```python
from build123d import *

# Parameters (mm, degrees)
CROQUIS1_R              = 3.645
SALIENTE_EXTRUIR1_DEPTH = 26.3


with BuildPart() as part:
    # Croquis1 → Saliente-Extruir1 (new body)
    with BuildSketch(Plane(origin=(0, 0, 0), x_dir=(0, 0, -1), z_dir=(1, 0, 0))):
        with BuildLine():
            Line((-14.240976213, -40.83193708), (-9.515976213, -40.83193708))
            Line((-9.515976213, -40.83193708), (-15.665976213, -34.68193708))
            Line((-15.665976213, -34.68193708), (-23.665976213, -34.68193708))
            Line((-23.665976213, -34.68193708), (-29.815976213, -40.83193708))
            Line((-29.815976213, -40.83193708), (-25.090976213, -40.83193708))
            ThreePointArc((-25.090976213, -40.83193708), (-23.665976213, -42.25693708), (-25.090976213, -43.68193708))
            Line((-25.090976213, -43.68193708), (-33.267411985, -43.655501308))
            ThreePointArc((-33.267411985, -43.655501308), (-34.256346235, -43.245871329), (-34.665976213, -42.25693708))
            Line((-34.665976213, -42.25693708), (-34.665976213, -34.10693708))
            ThreePointArc((-34.665976213, -34.10693708), (-33.267411985, -32.708372853), (-31.868847758, -34.10693708))
            Line((-31.868847758, -34.10693708), (-31.868847758, -38.83193708))
            Line((-31.868847758, -38.83193708), (-25.718847758, -32.68193708))
            Line((-25.718847758, -32.68193708), (-25.718847758, -24.68193708))
            Line((-25.718847758, -24.68193708), (-31.868847758, -18.53193708))
            Line((-31.868847758, -18.53193708), (-31.868847758, -23.25693708))
            ThreePointArc((-31.868847758, -23.25693708), (-33.293847758, -24.68193708), (-34.718847758, -23.25693708))
            Line((-34.718847758, -23.25693708), (-34.718847758, -15.10698367))
            ThreePointArc((-34.718847758, -15.10698367), (-34.301474921, -14.099356507), (-33.293847758, -13.68198367))
            Line((-33.293847758, -13.68198367), (-25.143847758, -13.68198367))
            ThreePointArc((-25.143847758, -13.68198367), (-23.718847758, -15.10698367), (-25.143847758, -16.53198367))
            Line((-25.143847758, -16.53198367), (-29.868847758, -16.53198367))
            Line((-29.868847758, -16.53198367), (-23.718847758, -22.68198367))
            Line((-23.718847758, -22.68198367), (-15.718847758, -22.68198367))
            Line((-15.718847758, -22.68198367), (-9.568847758, -16.53198367))
            Line((-9.568847758, -16.53198367), (-14.293847758, -16.53198367))
            ThreePointArc((-14.293847758, -16.53198367), (-15.718847758, -15.10698367), (-14.293847758, -13.68198367))
            Line((-14.293847758, -13.68198367), (-6.143847758, -13.68198367))
            ThreePointArc((-6.143847758, -13.68198367), (-5.136220595, -14.099356507), (-4.718847758, -15.10698367))
            Line((-4.718847758, -15.10698367), (-4.718847758, -23.153239985))
            ThreePointArc((-4.718847758, -23.153239985), (-6.143847758, -24.578239985), (-7.568847758, -23.153239985))
            Line((-7.568847758, -23.153239985), (-7.568847758, -18.53198367))
            Line((-7.568847758, -18.53198367), (-13.718847758, -24.68198367))
            Line((-13.718847758, -24.68198367), (-13.718847758, -32.68198367))
            Line((-13.718847758, -32.68198367), (-7.568847758, -38.83198367))
            Line((-7.568847758, -38.83198367), (-7.568847758, -34.003239985))
            ThreePointArc((-7.568847758, -34.003239985), (-6.143847758, -32.578239985), (-4.718847758, -34.003239985))
            Line((-4.718847758, -34.003239985), (-4.718847758, -42.25693708))
            ThreePointArc((-4.718847758, -42.25693708), (-5.136220595, -43.264564244), (-6.143847758, -43.68193708))
            Line((-6.143847758, -43.68193708), (-14.240976213, -43.68193708))
            ThreePointArc((-14.240976213, -43.68193708), (-15.665976213, -42.25693708), (-14.240976213, -40.83193708))
        make_face()
        with Locations((-19.665976213, -28.68193708)):
            Circle(CROQUIS1_R, mode=Mode.SUBTRACT)
    extrude(amount=SALIENTE_EXTRUIR1_DEPTH)


solid = part.part
```
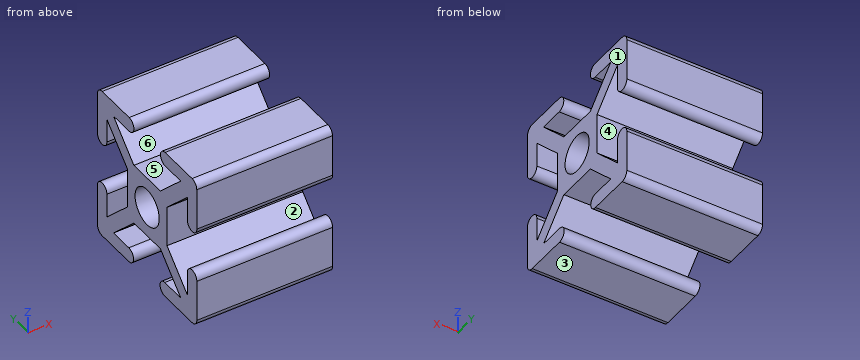
Build history of the part. All positions in model axes, mm. Face numbers are marked on the shaded views. A direction names the side the tool comes from. Round coordinates to 2 decimals unless told otherwise and drop trailing zeros. Loops run counter-clockwise (first coordinate to the right, second up) from the corner with the lowest first, then second, coordinate; pieces in that order, holes last.
Item 1: Drill centre lines: line 1 along Y through (x, z) = (7.5, 26); line 2 along Y through (x, z) = (10.75, 25); line 3 along Z through (x, y) = (12.25, -20.5). Where is each one in solid material? Low to high.
Item 2: Which spindle directions (+Z, -Z, +X, -X, +Y, -Y) get a long thin tool onto all of the face, cutting with end or side? Do the marked faces 4, 5 and 6. Say none if no direction does.
Item 3: Saw through at D-D (z = 27). List the corners of the cut face in (x, y), then the cut area to 3 significant figures.
Item 4: Saw through at A-A (y = -35.25). List the corners of the cut face in (x, z), then the cut area to 3 significant figures.
Item 5: Saw through at B-B (z = 15). List the corners of the cut face in (x, y).
Item 6: Saw through at C-C (z = 20.5). List the corners of the cut face in (x, y).
Item 7: Pin check, flat tips, straight feed: P1, Ø2.5, axis at x = 13, z = 27, coming from the -Y side; P2, Ø2.5, axis at x = 9.5, y = -38, coming from the +Z side; P3, Ø4, axis at x = 15, z = 20.5, coming from the -Y side. Stop position of each tip, or through.
Item 8: Two-plate mould, pull along Z, no slides. Class the marked faces 1, 2 and 3: released by +Z, released by -Z, zero draft, split by the parting line, or undercut.
Worked answers:
1. line 1: y = -43.68 to -40.83, -37.02 to -32.96, -24.4 to -20.4, -16.53 to -13.68
1. line 2: y = -43.68 to -40.83, -36.02 to -21.4, -16.52 to -13.69
1. line 3: z = 4.72 to 7.57, 9.54 to 13.54, 25.9 to 29.9, 31.87 to 34.72
2. face 4: +X, -X, +Y
2. face 5: +Z, +X, -X
2. face 6: +X, -X
3. outline: (0, -43.68) - (26.3, -43.68) - (26.3, -40.83) - (0, -40.83) - close; (0, -38.02) - (26.3, -38.02) - (26.3, -33.96) - (0, -33.96) - close; (0, -23.4) - (26.3, -23.4) - (26.3, -19.4) - (0, -19.4) - close; (0, -16.53) - (26.3, -16.53) - (26.3, -13.68) - (0, -13.68) - close
3. area: 362 mm2
4. outline: (0, 4.72) - (26.3, 4.72) - (26.3, 7.57) - (0, 7.57) - close; (0, 11.15) - (26.3, 11.15) - (26.3, 15.1) - (0, 15.1) - close; (0, 24.23) - (26.3, 24.23) - (26.3, 28.29) - (0, 28.29) - close; (0, 31.87) - (26.3, 31.87) - (26.3, 34.67) - (0, 34.67) - close
4. area: 359 mm2
5. outline: (0, -43.46) - (26.3, -43.46) - (26.3, -41.05) - (0, -41.05) - close; (0, -35.35) - (26.3, -35.35) - (26.3, -21.96) - (0, -21.96) - close; (0, -16.34) - (26.3, -16.34) - (26.3, -13.87) - (0, -13.87) - close
6. outline: (0, -34.68) - (26.3, -34.68) - (26.3, -32.23) - (0, -32.23) - close; (0, -25.13) - (26.3, -25.13) - (26.3, -22.68) - (0, -22.68) - close
7. P1: stops at y = -43.68
7. P2: stops at z = 34.67
7. P3: stops at y = -34.68
8. face 1: zero draft
8. face 2: undercut
8. face 3: released by -Z
